Verification items for this drawing (mm, ordinates from the low corner). Give positions to 0.01 mm unless a question says otherwise; leave off trailing zeros. Loops run counter-clockwise (first coordinate to the right, second up) from the corner with the lowest first, then second, coordinate; pieces in that order, holes last. Notation, with made-up numbers: (61.5, 54.5) -> (79.5, 54.5) arc R21 cw to (79.5, 88.5) -> close; hole circle Ø5 at (81, -32). An arc over 180 degrees is marked (long way). Write item = value, one per line.
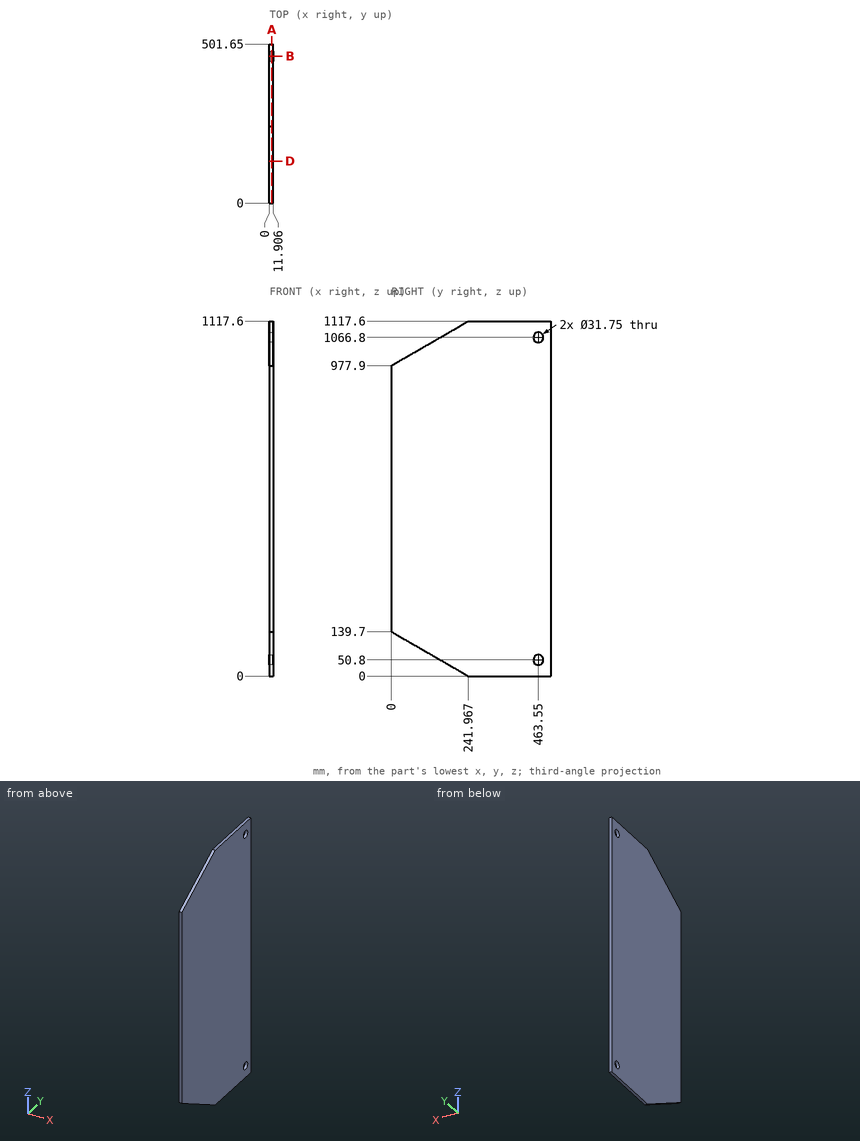
Item 1: Thickness scan on L1, parallel to Z at x = 1, y = 477 (1 decimal); L2, parallel to Z at x = 7.25, y = 210 (1 decimal); L3, parallel to Z at x = 5.75, y = 111 (1 decimal). Record the ranges inside material, lowest first. Write a range as [from, to].
Answer:
L1 = [0, 42.4], [59.2, 1058.4], [1075.2, 1117.6]
L2 = [18.5, 1099.1]
L3 = [75.6, 1042]
Item 2: Section check D-D, the plane y = 133. Record the cut outline in (x, z), plus the area to 3 significant figures.
Answer:
outline = (0, 62.91) -> (11.91, 62.91) -> (11.91, 1054.69) -> (0, 1054.69) -> close
area = 11,800 mm^2
Item 3: Section check B-B, the plane y = 463.55. Record the cut outline in (x, z) (1 decimal).
Answer:
outline = (0, 0) -> (11.9, 0) -> (11.9, 34.9) -> (0, 34.9) -> close; (0, 66.7) -> (11.9, 66.7) -> (11.9, 1050.9) -> (0, 1050.9) -> close; (0, 1082.7) -> (11.9, 1082.7) -> (11.9, 1117.6) -> (0, 1117.6) -> close
Item 4: Section check A-A, the plane x = 7.5. Give the number of separate pieces and of enclosed holes in the cut face, plus the area to 3 significant figures.
Answer:
separate_pieces = 1
enclosed_holes = 2
area = 525,000 mm^2
